For this review, use the dimensioned drawing (mm, ordinates from the lowest corner) and the shaded views. A direction names the side the tool comes from. Round coordinates to 2 decimals unless told otherwise and drop trailing zeros. Order: outer loops, then holes, each group sorted by start corner. A loop starts at its lowest first (then second) coordinate and runs counter-clockwise, first axis right, second up. Notation, with made-up numbers: (-33.75, -16.75) - (23.25, -16.75) arc R16 cw to (23.25, -12.75) - close; hole circle Ø5 at (-37, 57). An arc over 180 degrees is marked (long way). Write each question's results on one line, items separated by ' | '. Start each with the question number.
(1) For L1, parallel to Y at x = 70.5, z = 8; L2, parallel to Z at x = 89.5, y = 30, list the stretches that pass through material, from the lowest coordinate up. Write a range as from..to.
(2) Take a section at A-A, the plane x = 17.5. Give the boundary of the cut face in (y, z).
(3) For the marked faces 5 and 6, list the 3-axis set-ups (+Z, -Z, +X, -X, +Y, -Y) from which the entire face can be reached by the end or side of a thin tool; tool diameter is ignored.
(4) Take a section at C-C, the plane z = 7. Give the number of separate pieces and of enclosed holes in the cut face, plus the area to 3 significant figures.
(5) Draft analysis for pull direction Y (two halves, no side actions). For the marked faces 1, 2, 3 and 4, state which applies: pulls with the +Y half, pulls with the -Y half, needs draft (parallel to the pull), parting line crosses it, or undercut.
(6) Insertion check: pin 1 Ø19 at (x, y) = (23.5, 27.5) entering from +Z. The pin has a flat end and moves straight along its axis. Give the tip position at first contact, or say it passes through.
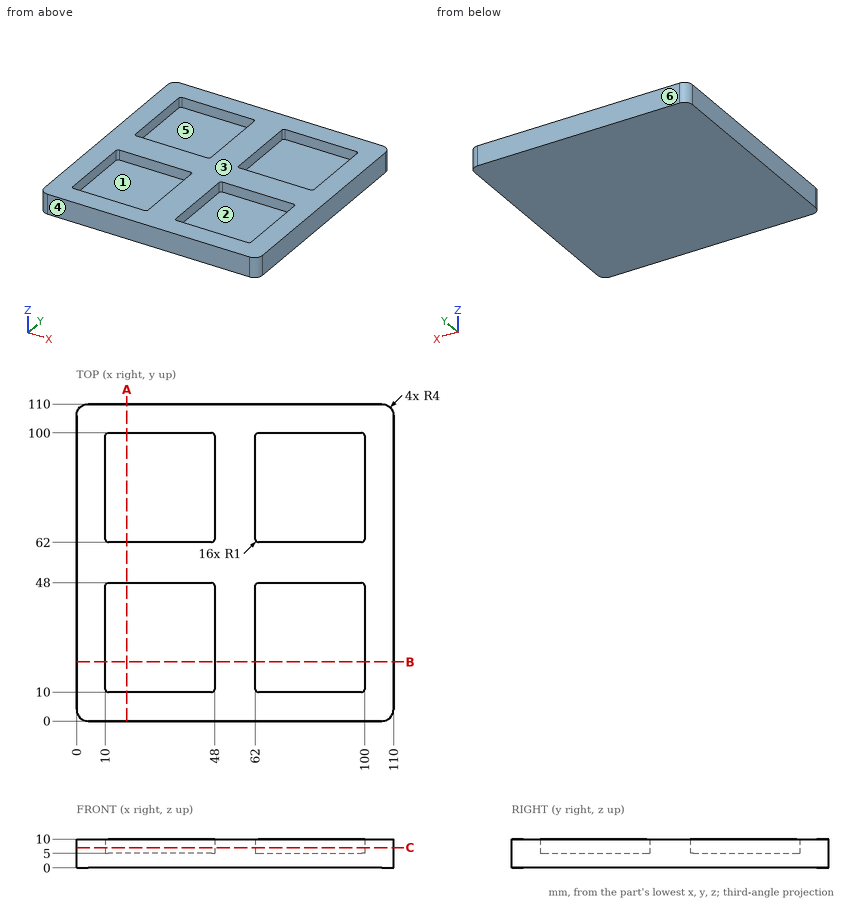
Results below:
1) L1: y = 0..10, 48..62, 100..110 | L2: z = 0..5
2) outline: (0, 0) - (110, 0) - (110, 10) - (100, 10) - (100, 5) - (62, 5) - (62, 10) - (48, 10) - (48, 5) - (10, 5) - (10, 10) - (0, 10) - close
3) face 5: +Z | face 6: +Z, -Z, +X, -X, +Y
4) separate pieces: 1 | enclosed holes: 4 | area: 6,310 mm^2
5) face 1: undercut | face 2: undercut | face 3: needs draft | face 4: pulls with the -Y half
6) pin 1: stops at z = 5
